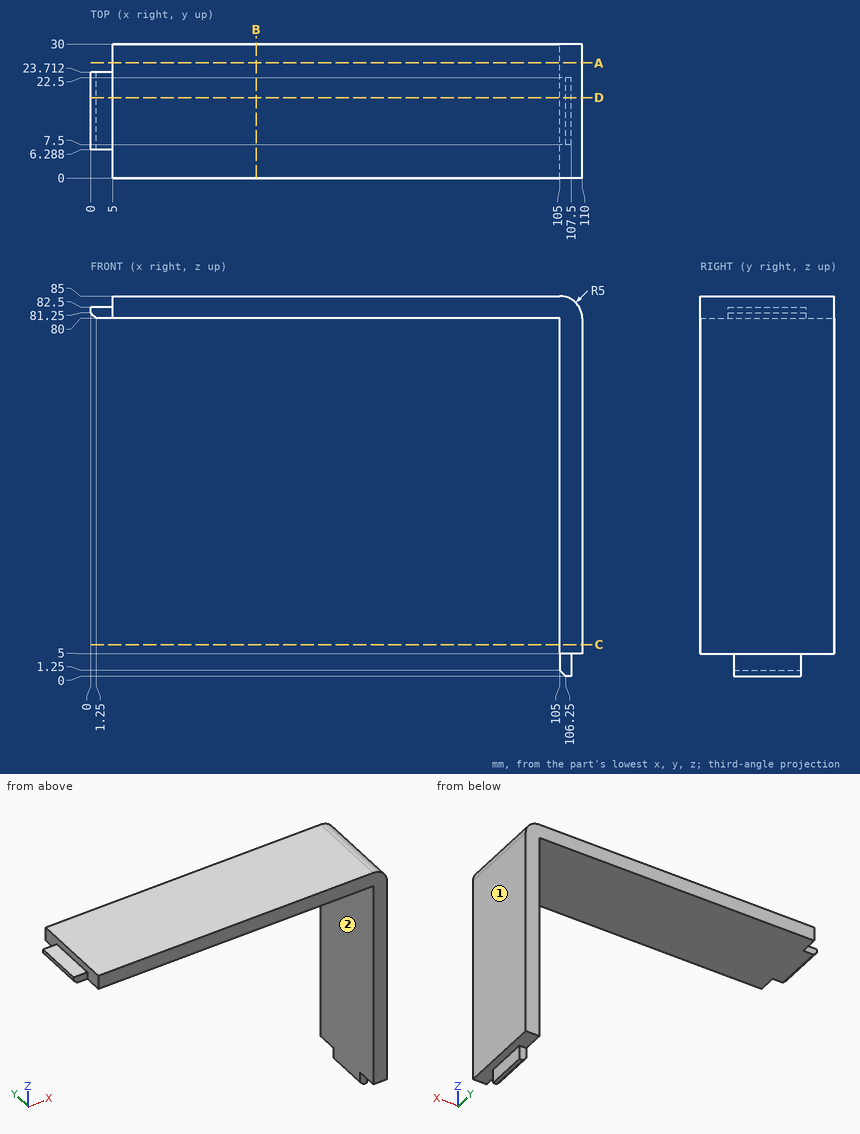
Can you work these out from the drawing? Everything is in mm from the part's minimum corner. A direction names the side the tool comes from. Coordinates: 2 decimals unless noted, no trailing zeros. Loops run counter-clockwise (first coordinate to the right, second up) from the corner with the lowest first, then second, coordinate; pieces in that order, holes last.
1) Will these pins go through, and if not, where does the flat tip stop? pin 1 Ø1.2 at (x, z) = (3.5, 81.5) entering from -Y; pin 2 Ø5 at (y, z) = (9.5, 50) entering from -X; pin 3 Ø1 at (x, y) = (43.5, 10) entering from -Z.
Reported:
pin 1: stops at y = 6.29
pin 2: stops at x = 105
pin 3: stops at z = 80
2) Which directions (+Z, -Z, +X, -X, +Y, -Y) give clear straight access to the entire face, cutting with the end or side of a thin tool? Please do the marked faces 1 and 2.
Reported:
face 1: +Z, -Z, +X, +Y, -Y
face 2: -Z, -X, +Y, -Y
3) Imagine slicing it at B-B (x = 37). List the corners of the cut face in (y, z) for me, and give its area (3 significant figures).
Reported:
outline: (0, 80) - (30, 80) - (30, 85) - (0, 85) - close
area: 150 mm2
4) Please list where these lines run through material, in increasing order: line 1 along Z through (x, y) = (5.5, 27); line 2 along X through (y, z) = (14.5, 42).
Reported:
line 1: z = 80 to 85
line 2: x = 105 to 110
5) Imagine slicing it at A-A (y = 25.75). List the corners of the cut face in (x, z) for me.
Reported:
outline: (5, 80) - (105, 80) - (105, 5) - (110, 5) - (110, 80) arc R5 ccw to (105, 85) - (5, 85) - close
6) Imagine slicing it at D-D (y = 18). List the corners of the cut face in (x, z) for me, and give its area (3 significant figures).
Reported:
outline: (0, 81.25) - (1.25, 80) - (105, 80) - (105, 1.25) - (106.25, 0) - (107.5, 0) - (107.5, 5) - (110, 5) - (110, 80) arc R5 ccw to (105, 85) - (5, 85) - (5, 82.5) - (0, 82.5) - close
area: 918 mm2
7) Imagine slicing it at C-C (z = 7). List the corners of the cut face in (x, y) for me, and give its area (3 significant figures).
Reported:
outline: (105, 0) - (110, 0) - (110, 30) - (105, 30) - close
area: 150 mm2
